Work out the finished part from the listing and answer in its coordinate system (mm). A direction names the side the tool comes from. Give positions to 0.01 mm unless a question says otherwise; leave off trailing zeros. Order: outer loops, then holes, each group sorted by start corner. A loop starts at its lowest first (then second) coordinate and runs counter-clockwise, first axis right, second up. Notation, with made-up numbers: M -30,39.5 L 25,39.5 A17 cw 25,44.5 Z; hole C -10.5,88.5 d9. An arc over 180 degrees is marked long. One line per item, written item: value.
from build123d import *

# Parameters (mm, degrees)
F1_DEPTH = 12
F2_R     = 2.5
F3_DEPTH = 4
F4_R     = 3
F5_DEPTH = 12


with BuildPart() as f1:
    # F0 (on Front) → F1 (new body)
    with BuildSketch(Plane.XZ):
        Polygon((18.994565, 9.5), (-26.005435, 9.5), (-26.005435, -2.5), (48.994565, -2.5), (48.994565, 0), align=None)
    extrude(amount=F1_DEPTH)

    # F2 (on face) → F3 (cut)
    with BuildSketch(Plane(origin=(0, 0, -2.5), x_dir=(1, 0, 0), z_dir=(0, 0, -1))):
        with Locations((-18.005435, 6)):
            Circle(F2_R)
    extrude(amount=-F3_DEPTH, mode=Mode.SUBTRACT)

    # F4 (on face) → F5 (cut)
    with BuildSketch(Plane(origin=(0, 0, -2.5), x_dir=(1, 0, 0), z_dir=(0, 0, -1))):
        with Locations((10.994565, 6)):
            Circle(F4_R)
    extrude(amount=-F5_DEPTH, mode=Mode.SUBTRACT)


solid = f1.part
(1) Section A-A, the plane y = -6 is taken. Give the vertices of the cut face in (x, z).
Findings:
outline: M -26.01,-2.5 L -20.51,-2.5 L -20.51,1.5 L -15.51,1.5 L -15.51,-2.5 L 7.99,-2.5 L 7.99,9.5 L -26.01,9.5 Z; M 13.99,-2.5 L 48.99,-2.5 L 48.99,0 L 18.99,9.5 L 13.99,9.5 Z
(2) Given P1, Ø5.5, axis at x = 10.99, y = -6, coming from the +Z side, flat-ended and moving along its own axis, determine where the tip first touches the part or whether it passes through.
Findings:
P1: passes through
(3) Find the intervals of material crossed by probe 1 along X at (y, z) = (-6, -0.8); probe 2 along Z at (x, y) = (19, -4.25); probe 3 along Z at (x, y) = (20, -6.5), in increasing order. Write a range as from..to.
Findings:
probe 1: x = -26.01..-20.51, -15.51..7.99, 13.99..48.99
probe 2: z = -2.5..9.5
probe 3: z = -2.5..9.18
(4) Section D-D, the plane x = -19.5 is taken. Give the vertices of the cut face in (y, z).
Findings:
outline: M -12,-2.5 L -8,-2.5 L -8,1.5 L -4,1.5 L -4,-2.5 L 0,-2.5 L 0,9.5 L -12,9.5 Z
(5) Section C-C, the plane x = 9.5 is taken. Give the vertices of the cut face in (y, z), then the cut area to 3 significant figures.
Findings:
outline: M -12,-2.5 L -8.6,-2.5 L -8.6,9.5 L -12,9.5 Z; M -3.4,-2.5 L 0,-2.5 L 0,9.5 L -3.4,9.5 Z
area: 81.6 mm^2
(6) Determine the mould class of faces 3 (the flat face through (48.995, -6, -1)), 4 (the flat face through (3, 0, 4)), 5 (the cylindrical face through (13.766, -4.851, 3.416)) for opening direction Y: pulls with the +Y half, pulls with the -Y half, needs draft (parallel to the pull), parting line crosses it, or undercut.
Findings:
face 3: needs draft
face 4: pulls with the +Y half
face 5: undercut
(7) Which of the six approach directions +Z, -Z, +X, -X, +Y, -Y give full straight-line access (tool end or side, diameter ignored) to faces 1 (the flat face through (-3, -6, 9.5)), 2 (the cylindrical face through (-15.62, -6.75, -0.53))?
Findings:
face 1: +Z, +X, -X, +Y, -Y
face 2: -Z
(8) Section B-B, the plane z = 2.25 is taken. Give the vertices of the cut face in (x, y), then the cut area to 3 significant figures.
Findings:
outline: M -26.01,-12 L 41.89,-12 L 41.89,0 L -26.01,0 Z; hole C 10.99,-6 d6
area: 786 mm^2
